Can you work these out from the model? Positions are in its coordinate system, mm. Coordinates: 2 decimals unless noted, no trailing zeros. Order: outer loops, then holes, each group sorted by start corner. A loop starts at its lowest first (then second) coordinate and runs counter-clockwise, first axis right, second up. Notation, with made-up numbers: (69, 8) -> (104, 8) arc R29 cw to (104, 43) -> close; hole circle Ø2 at (57.5, -14.75). An arc over 180 degrees is marked (long way). Answer as CSV lines item,"result".
Autodesk Fusion 360 part; units mm, degrees
sketch "Sketch1" plane through (0, 0, 0) normal (1, 0, 0) x (0, 1, 0)
  circle A0 centre (0, 0) radius 9.332
  line L0 (-0.293, -15.7817) -> (50.7077, -15.7817)
  line L1 (74.0537, -2.44) -> (108.9435, 56.7771)
  line L2 (-8.9747, 12.9847) -> (94.4391, 71.534)
  arc A1 (50.7077, -15.7817) -> (74.0537, -2.44) centre (50.7077, 11.3152) ccw
  arc A2 (-6.5163, 14.3766) -> (0.293, -15.7817) centre (0, 0) ccw
  arc A3 (108.9435, 56.7771) -> (94.4391, 71.534) centre (99.7158, 62.2139) ccw
  circle A4 centre (99.7158, 62.2139) radius 6.0013
  dimension "d1" = 27.0969
  dimension "d3" = 15.7844
  dimension "d4" = 18.6641
  dimension "d5" = 12.0025
  dimension "d6" = 10.7102
  dimension "d7" = 59.494
  dimension "d8" = 29.517
  dimension "d12" = 77.9956
  dimension "d13" = 99.7158
  dimension "d16" = 118.8379
sketch "Sketch3" plane through (0, 0, 0) normal (1, 0, 0) x (0, 1, 0)
  line L0 (81.0105, 50.2421) -> (22.4827, 17.1057)
  line L1 (22.4827, 17.1057) -> (22.4827, -4.1678)
  line L2 (22.4827, -4.1678) -> (34.4677, -4.1678)
  line L3 (71.7994, 17.1664) -> (88.731, 45.9038)
  line L4 (88.731, 45.9038) -> (81.0105, 50.2421)
  arc A0 (34.4677, -4.1678) -> (71.7994, 17.1664) centre (34.4677, 39.1617) ccw
  dimension "d17" = 43.3295
extrude "Extrude1" add sketch "Sketch1" against normal blind 49.171 contours L0 L1 L2 A1 A2 A3
Q1. Imagine slicing it at C-C (x = -20). List the corners of the cut face in (y, z) for me.
Solution:
outline,"(-8.97, 12.98) arc R15.78 ccw to (-0.29, -15.78) -> (50.71, -15.78) arc R27.1 ccw to (74.05, -2.44) -> (108.94, 56.78) arc R10.71 ccw to (94.44, 71.53) -> close; hole circle Ø18.66 at (0, 0); hole circle Ø12 at (99.72, 62.21)"
Q2. Imagine slicing it at A-A (z = -7.5). List the corners of the cut face in (x, y) for me, and give its area (3 significant figures).
Solution:
outline,"(-49.17, -13.89) -> (0, -13.89) -> (0, -5.55) -> (-49.17, -5.55) -> close; (-49.17, 5.55) -> (0, 5.55) -> (0, 70.21) -> (-49.17, 70.21) -> close"
area,"3,590 mm2"
Q3. Imagine slicing it at B-B (y = -4.5). List the corners of the cut face in (x, z) for me, and give its area (3 significant figures).
Solution:
outline,"(-49.17, -15.13) -> (0, -15.13) -> (0, -8.18) -> (-49.17, -8.18) -> close; (-49.17, 8.18) -> (0, 8.18) -> (0, 15.52) -> (-49.17, 15.52) -> close"
area,"703 mm2"
Q4. We'd pull the mould along Z, two halves only. Please class faces 1 (the cylindrical face through (-24.24, -15.19, -4.29)), 2 (the cylindrical face through (-24.241, 94.953, 58.562)), 3 (the cylindrical face through (-24.24, 63.98, -12.31)): pulls with the +Z half, pulls with the -Z half, needs draft (parallel to the pull), parting line crosses it, or undercut.
Solution:
face 1,"parting line crosses it"
face 2,"undercut"
face 3,"pulls with the -Z half"
Q5. If I drill on line 1 (Z direction, x = -25, y = 105); line 2 (Z direction, x = -30, y = 0); line 3 (Y direction, x = -41.5, z = 61), over which ranges is the centre line in solid material (lowest first)?
Solution:
line 1,"50.08 to 59.37, 65.06 to 71.53"
line 2,"-15.78 to -9.33, 9.33 to 18.07"
line 3,"75.83 to 93.84, 105.59 to 110.36"
Q6. Imagine slicing it at D-D (z = 22.5). List the corners of the cut face in (x, y) for me.
Solution:
outline,"(-49.17, 7.83) -> (0, 7.83) -> (0, 88.75) -> (-49.17, 88.75) -> close"
Q7. For P1, Ø1.5, axis at x = -15, y = 88.5, coming from the +Z side; P2, Ø2, axis at x = -18, y = 90.5, coming from the -Z side; P3, Ø2, axis at x = -36.5, z = 36.5, coming from the -Y side, each with a flat end and sliding along its axis, tell me the tip position at first contact or that it passes through.
Solution:
P1,"z = 68.6"
P2,"z = 23.78"
P3,"y = 30.79"
